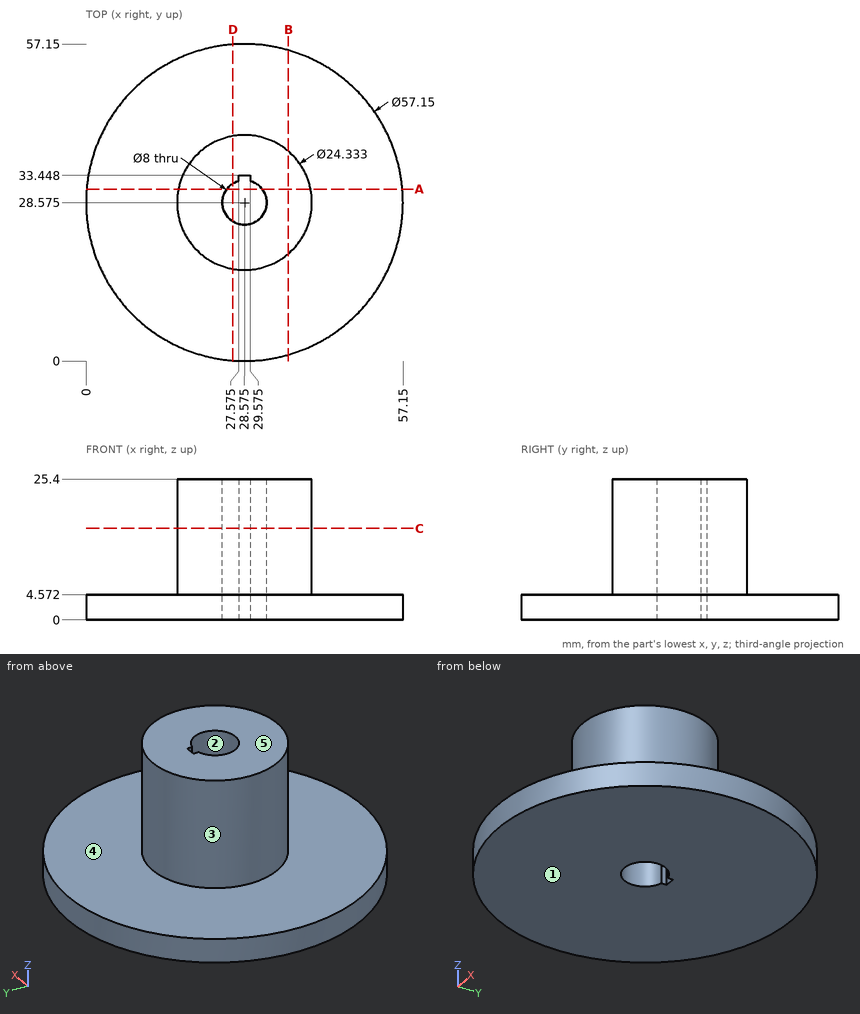
Can you work these out from the drawing? Everything is in mm from the part's minimum corner. A direction names the side the tool comes from. Round coordinates to 2 decimals unless told otherwise and drop trailing zeros. Write each loop counter-clockwise with the first axis right and the second up, starting at its lowest first coordinate (ties: lowest second). Pieces come first, ordered by that corner, then holes. Notation, with made-up numbers: (9.25, 68.5) - (17.25, 68.5) arc R25 ccw to (17.25, 89.5) - close; hole circle Ø6 at (35.5, 8.5). An arc over 180 degrees is marked (long way). Put each result on its own line as item: value. Start each with the question number.
(1) I need wall thicknesses on probe 1 along Z at (x, y) = (40, 17); probe 2 along Y at (x, z) = (28, 19.75); probe 3 along X at (y, z) = (32, 10.5). Which ranges of each line are inside material? Lowest first, please.
(2) For the marked faces 4 and 5, which set-ups out of +Z, -Z, +X, -X, +Y, -Y let a thin tool reach every point of the face, with its end or its side?
(3) I want a section at C-C, the plane z = 16.5. Please give me the cut outline in (x, y) (1 decimal).
(4) Thinking about a two-plate mould opening in Y: for the marked faces 1, 2 and 3, which applies, released by +Y, released by -Y, zero draft, split by the parting line, or undercut?
(5) I want a section at A-A, the plane y = 31. Please give me the cut outline in (x, z), plus the area to 3 significant figures.
(6) I want a section at B-B, the plane x = 36.5. Please give me the cut outline in (y, z).
(7) Will these pins go through, and if not, where does the flat tip stop? pin 1 (0.6 mm diameter, centred on x = 29, z = 11.5, fed in from -Y); pin 2 (5 mm diameter, centred on x = 48, y = 34.5, fed in from +Z); pin 3 (1 mm diameter, centred on y = 15, z = 3.5, fed in from -X).
(8) I want a section at D-D, the plane x = 26.5. Please give me the cut outline in (y, z) (1 decimal).
Here are the results:
1. probe 1: z = 0 to 4.57
1. probe 2: y = 16.42 to 24.62, 33.45 to 40.73
1. probe 3: x = 16.9 to 26.51, 30.64 to 40.25
2. face 4: +Z
2. face 5: +Z, +X, -X, +Y, -Y
3. outline: circle Ø24.3 at (28.6, 28.6); hole (27.6, 32.4) arc R4 ccw (long way) to (29.6, 32.4) - (29.6, 33.4) - (27.6, 33.4) - close
4. face 1: zero draft
4. face 2: undercut
4. face 3: split by the parting line
5. outline: (0.1, 0) - (25.39, 0) - (25.39, 25.4) - (16.65, 25.4) - (16.65, 4.57) - (0.1, 4.57) - close; (31.76, 0) - (57.05, 0) - (57.05, 4.57) - (40.5, 4.57) - (40.5, 25.4) - (31.76, 25.4) - close
5. area: 595 mm^2
6. outline: (1.12, 0) - (56.03, 0) - (56.03, 4.57) - (37.81, 4.57) - (37.81, 25.4) - (19.34, 25.4) - (19.34, 4.57) - (1.12, 4.57) - close
7. pin 1: stops at y = 16.41
7. pin 2: stops at z = 4.57
7. pin 3: stops at x = 3.17
8. outline: (0.1, 0) - (25.2, 0) - (25.2, 25.4) - (16.6, 25.4) - (16.6, 4.6) - (0.1, 4.6) - close; (32, 0) - (57.1, 0) - (57.1, 4.6) - (40.6, 4.6) - (40.6, 25.4) - (32, 25.4) - close
